Input: part model. Units: mm. Frame: model coordinates. A direction names the side the tool comes from. Give positions to 0.01 mm unless a question says otherwise; leave off trailing zeros. Write each loop counter-clockwise with the first axis right and the second up, starting at its lowest first coordinate (ties: lowest second). Pieces come first, ordered by that corner, then holes. Notation, with made-up numbers: (74.25, 26.5) -> (101.25, 26.5) arc R25 ccw to (101.25, 40.5) -> close; hole circle Ø11 at (23.25, -7). An arc over 180 degrees is marked (long way). Return JSON: item names as keys, results as strings. Group by question number.
Item 1: Set-up query: faces 5 (the face through (0, 0, 0)), 6 (the face through (12.7, 3, -9)). Return all of +Z, -Z, +X, -X, +Y, -Y with unobstructed straight access to the full face (end or side cutting, diameter ignored); none if empty.
Item 2: Section A-A, the plane z = -7. Return loops of the section in (x, y).
Item 3: Pin query (flat end, axial travel): P1, Ø4, axis at x = 12, z = 9, coming from the -Y side; P2, Ø3, axis at x = 21.5, y = 4.5, coming from the -Z side. Return the tip coordinate at first contact, or that it passes through.
Item 4: Line query: line 1 (X direction, y = 5.25, z = -11.25); line 2 (Z direction, x = -10.5, y = 6). Output: solid intervals per line, ascending. Write a range as [from, to].
Item 5: Section B-B, the plane y = 4.25. Return loops of the section in (x, z).
Item 6: Mould query, pull axis X, two halves, no side actions, for faces 1 (the face through (31.75, 3, 0)), 2 (the face through (19.05, 3, -9)), 3 (the face through (0, 3, 12.7)), 4 (the face through (-31.75, 3, 0)). Classes: released by +X, released by -X, zero draft, split by the parting line, or undercut.
Item 7: Section C-C, the plane x = -24.5. Return loops of the section in (y, z).
from build123d import *

# Parameters (mm, degrees)
SKETCH1_W           = 6.35
SKETCH1_H           = 6.35
BOSS_EXTRUDE1_DEPTH = 6.35


with BuildPart() as part:
    # Sketch1 → Boss-Extrude1 (new body)
    with BuildSketch(Plane(origin=(0, 0, 0), x_dir=(1, 0, 0), z_dir=(0, 1, 0))):
        Polygon((-31.75, 12.7), (-31.75, -12.7), (31.75, -12.7), (31.75, 12.7), (25.4, 12.7), (25.4, 6.35), (19.05, 6.35), (12.7, 6.35), (-12.7, 6.35), (-19.05, 6.35), (-25.4, 6.35), (-25.4, 12.7), align=None)
        with Locations((-15.875, 9.525)):
            Rectangle(SKETCH1_W, SKETCH1_H)
        with Locations((15.875, 9.525)):
            Rectangle(SKETCH1_W, SKETCH1_H)
    extrude(amount=BOSS_EXTRUDE1_DEPTH)


solid = part.part
Answer below:
{
 "1": {"face 5": "+Z, -Z, +X, -X, -Y", "face 6": "-Z, +Y, -Y"},
 "2": {"outline": "(-31.75, 0) -> (-25.4, 0) -> (-25.4, 6.35) -> (-31.75, 6.35) -> close; (-19.05, 0) -> (-12.7, 0) -> (-12.7, 6.35) -> (-19.05, 6.35) -> close; (12.7, 0) -> (19.05, 0) -> (19.05, 6.35) -> (12.7, 6.35) -> close; (25.4, 0) -> (31.75, 0) -> (31.75, 6.35) -> (25.4, 6.35) -> close"},
 "3": {"P1": "stops at y = 0", "P2": "stops at z = -6.35"},
 "4": {"line 1": "x = [-31.75, -25.4], [-19.05, -12.7], [12.7, 19.05], [25.4, 31.75]", "line 2": "z = [-6.35, 12.7]"},
 "5": {"outline": "(-31.75, -12.7) -> (-25.4, -12.7) -> (-25.4, -6.35) -> (-19.05, -6.35) -> (-19.05, -12.7) -> (-12.7, -12.7) -> (-12.7, -6.35) -> (12.7, -6.35) -> (12.7, -12.7) -> (19.05, -12.7) -> (19.05, -6.35) -> (25.4, -6.35) -> (25.4, -12.7) -> (31.75, -12.7) -> (31.75, 12.7) -> (-31.75, 12.7) -> close"},
 "6": {"face 1": "released by +X", "face 2": "undercut", "face 3": "zero draft", "face 4": "released by -X"},
 "7": {"outline": "(0, -6.35) -> (6.35, -6.35) -> (6.35, 12.7) -> (0, 12.7) -> close"}
}
